For this review, take the finished solid that the model builds, in its own axes (mm). A direction names the side the tool comes from. Coordinates: 2 decimals unless noted, no trailing zeros. Order: outer loops, then holes, each group sorted by start corner. A loop starts at its lowest first (then second) coordinate and runs counter-clockwise, first axis right, second up.
Autodesk Inventor part; units mm, degrees
ref_plane "YZ Plane" through (0, 0, 0) normal (1, 0, 0) x (0, 1, 0)
ref_plane "XZ Plane" through (0, 0, 0) normal (0, 1, 0) x (-1, 0, 0)
ref_plane "XY Plane" through (0, 0, 0) normal (0, 0, 1) x (1, 0, 0)
sketch "Sketch1" plane through (0, 0, 0) normal (0, 1, 0) x (-1, 0, 0)
  line L0 (30, -30) -> (-30, -30)
  line L1 (-30, -30) -> (-30, 30)
  line L2 (-30, 30) -> (30, 30)
  line L3 (30, 30) -> (30, -30)
  line L4 (30, -30) -> (-30, 30) construction
  line L5 (-30, -30) -> (30, 30) construction
  point P0 (0, 0)
  dimension "d0" = 60
  dimension "d1" = 60
extrude "Extrusion1" add sketch "Sketch1" along normal blind 20
sketch "Sketch2" plane through (0, 0, 0) normal (0, -1, 0) x (1, 0, 0)
  circle A0 centre (0, 0) radius 27.5
  dimension "d4" = 55
extrude "Extrusion2" cut sketch "Sketch2" against normal blind 20
sketch "Sketch3" plane through (0, 0, 0) normal (0, -1, 0) x (1, 0, 0)
  circle A0 centre (0, 0) radius 30
  line L0 (-30, -30) -> (30, -30)
  line L1 (30, -30) -> (30, 30)
  line L2 (30, 30) -> (-30, 30)
  line L3 (-30, 30) -> (-30, -30)
  line L4 (-30, -30) -> (30, 30) construction
  line L5 (30, -30) -> (-30, 30) construction
extrude "Extrusion3" cut sketch "Sketch3" against normal blind 17 contours L1 L0 A0 | A0 L2 L1 | A0 L3 L2 | L0 L3 A0
sketch "Sketch4" plane through (0, 0, 0) normal (1, 0, 0) x (0, 1, 0)
  line L0 (0, 30) -> (0, -30)
  line L1 (0, -30.2901) -> (3, -30.2901)
  line L2 (3, -30.2901) -> (3, 30)
  line L3 (3, 30) -> (0, 30)
  line L4 (0, 30) -> (0, -30.2901)
  point P0 (0, 0)
  dimension "d9" = 3
extrude "Extrusion4" add sketch "Sketch4" along normal mid plane 60
sketch "Sketch5" plane through (0, 0, 0) normal (0, -1, 0) x (1, 0, 0)
  circle A0 centre (0, 0) radius 27.5
extrude "Extrusion5" cut sketch "Sketch5" against normal blind 60
sketch "Sketch6" plane through (0, 0, 0) normal (0, -1, 0) x (1, 0, 0)
  circle A0 centre (25, -25.2901) radius 2
  circle A1 centre (-25, -25.2901) radius 2
  circle A2 centre (-25, 25) radius 2
  circle A3 centre (25, 25) radius 2
  line L0 (30, 30) -> (30, -30.2901)
  line L1 (-30, 30) -> (30, 30)
  line L2 (30, -30.2901) -> (-30, -30.2901)
  line L3 (-30, -30.2901) -> (-30, 30)
  point P0 (0, 0)
  dimension "d14" = 4
  dimension "d15" = 4
  dimension "d16" = 4
  dimension "d17" = 4
  dimension "d18" = 5
  dimension "d19" = 5
  dimension "d20" = 5
  dimension "d21" = 5
  dimension "d22" = 5
  dimension "d23" = 5
  dimension "d24" = 5
  dimension "d25" = 5
extrude "Extrusion6" cut sketch "Sketch6" against normal blind 60 keep common part
properties part number "ventilator"
1. Clearance check with flat-ended pins moving along their axes: pin 1 Ø6 at (y, z) = (13.5, 12.5) entering from -X; pin 2 Ø6 at (y, z) = (10, 4.5) entering from -X; pin 3 Ø1 at (x, y) = (-3.5, 12) entering from +Z; pin 4 Ø9 at (x, z) = (14.5, -18.5) entering from +Y. State where each tip first meets the part, or that it passes through.
Answer below:
pin 1: stops at x = -28.46
pin 2: stops at x = -29.96
pin 3: stops at z = 29.85
pin 4: stops at y = 20
2. Machinability: for faces 1 (the face through (-24, 3, 23)), 2 (the face through (-23, 17, -23)), 3 (the face through (4, 3, -30)), 4 (the face through (23, 17, 24)), 5 (the face through (23, 17, -23)), which of the approach directions +Z, -Z, +X, -X, +Y, -Y give a long, thin tool a straight path to every point of the face, cutting with its end or side? Answer none if there is none.
Answer below:
face 1: +Z, -X
face 2: -Z, -X
face 3: -Z
face 4: +Z, +X
face 5: -Z, +X
3. To check wall thickness, follow L1, parallel to Z at x = -25, y = 18.8; L2, parallel to Z at x = -25, y = 2; L3, parallel to X at y = 14.25, z = -10. State the ranges of each line that lie inside material, in increasing order.
Answer below:
L1: z = -30 to -27.29, -23.29 to -11.46, 11.46 to 23, 27 to 30
L2: z = -30.29 to -27.29, -23.29 to -11.46, 11.46 to 23, 27 to 30
L3: x = -28.28 to -25.62, 25.62 to 28.28
4. Take a section at B-B, the plane z = -21. Give the boundary of the cut face in (x, y).
Answer below:
outline: (-30, 0) - (-17.76, 0) - (-17.76, 20) - (-30, 20) - (-30, 17) - (-21.42, 17) - (-21.42, 3) - (-30, 3) - close; (17.76, 0) - (30, 0) - (30, 3) - (21.42, 3) - (21.42, 17) - (30, 17) - (30, 20) - (17.76, 20) - close
5. Take a section at A-A, the plane x = 18.5. Give the boundary of the cut face in (y, z).
Answer below:
outline: (0, -30.29) - (3, -30.29) - (3, -23.62) - (17, -23.62) - (17, -30) - (20, -30) - (20, -20.35) - (0, -20.35) - close; (0, 20.35) - (20, 20.35) - (20, 30) - (17, 30) - (17, 23.62) - (3, 23.62) - (3, 30) - (0, 30) - close
6. The part is to be moulded in two halves that separate along Y. For faces 6 (the face through (24, 3, 23)), 7 (the face through (27, 0, -7)), 8 (the face through (0, 2, 30)), 9 (the face through (-29.97, 9.9, 1.32)), say which applies: +Y half, -Y half, draft (parallel to the pull), parting line (faces both ways), or undercut.
Answer below:
face 6: undercut
face 7: -Y half
face 8: draft
face 9: undercut
7. Take a section at C-C, the plane z = 25. Give the number of separate pieces and of enclosed holes in the cut face, plus the area to 3 significant figures.
Answer below:
separate pieces: 6
enclosed holes: 0
area: 318 mm2
